Answer from the drawing. Dimensions are ordinates in mm from the lowest x, y and z of the part. A direction names the side the tool comes from. Coordinates: 2 decimals unless noted, no trailing zeros. Order: outer loops, then holes, each group sorted by start corner. A loop starts at its lowest first (then second) coordinate and runs counter-clockwise, first axis right, second up. Notation, with made-up numbers: M 54.5,6.25 L 81.5,6.25 A22 ccw 81.5,37.25 Z; hole C -6.5,13.5 d8. An arc over 180 degrees is marked long. One line per question, with ' | ' between items. Start each with the question number.
1) The mould has two halves that part along X. Classify the marked faces 3, 4, 5 and 6: +X half, -X half, draft (parallel to the pull), parting line (faces both ways), or undercut.
2) Given P1, Ø1.5, axis at y = 1.5, z = 5, coming from the -X side; P2, Ø1.1, axis at y = 1.5, z = 7.5, coming from the +X side (1 decimal); P3, Ø1.5, axis at y = 8, z = 9, coming from the +X side, each flat-ended and moving along its own axis, determine where each tip first touches the part or whether it passes through.
3) Find section D-D, the plane y = 8.5. Write down the section's boundary in (x, z).
4) Find section A-A, the plane x = 5.75. Write down the section's boundary in (y, z) (1 decimal).
5) Consider probe 1 along X at (y, z) = (5, 7); probe 2 along X at (y, z) = (7.5, 8.75) (1 decimal); probe 3 along X at (y, z) = (8.5, 1.25) (1 decimal). Determine where each line is inside the solid, lowest interval first.
6) Find section B-B, the plane y = 5.5. Write down the section's boundary in (x, z).
7) A tool of negligible diameter and unlimited length cuts with its end or side. For the marked faces 1 and 2, from which of +Z, -Z, +X, -X, +Y, -Y can it reach the whole face along a straight path? Write none if from no direction.
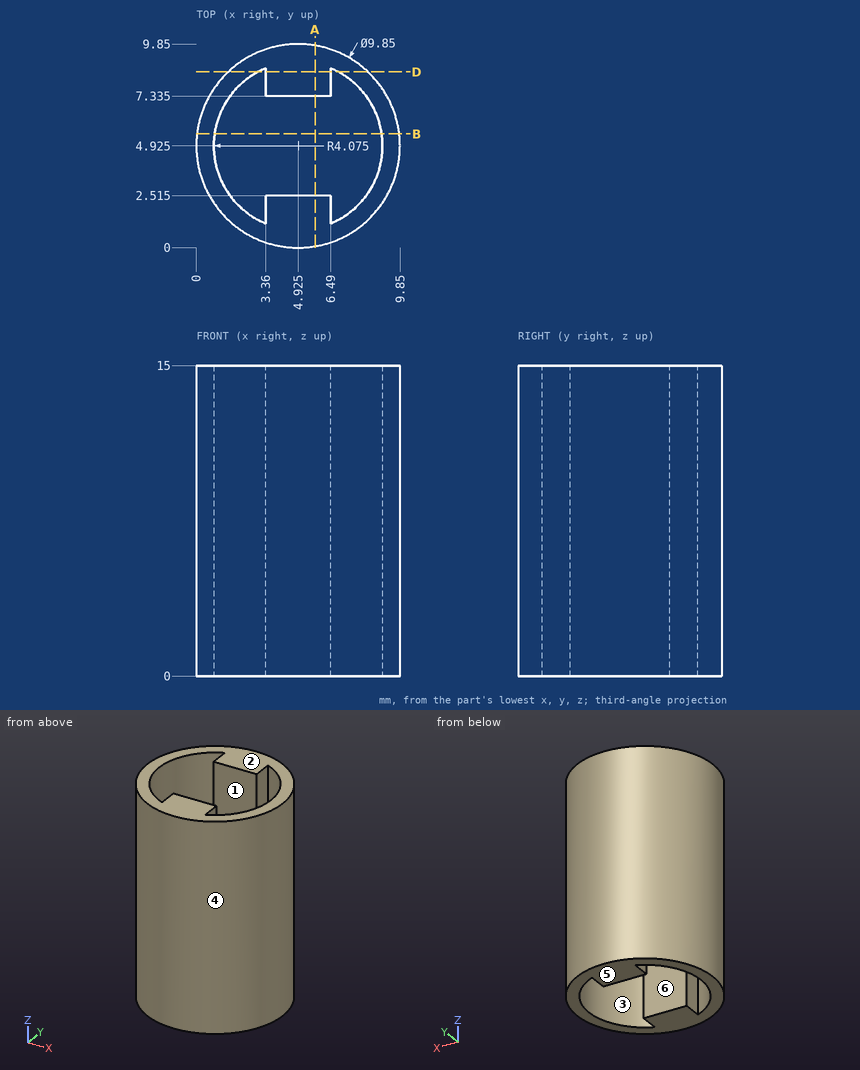
Report:
1) face 3: undercut | face 4: parting line | face 5: draft | face 6: undercut
2) P1: stops at x = 0.79 | P2: stops at x = 8.9 | P3: stops at x = 9.27
3) outline: M 1.54,0 L 2.97,0 L 2.97,15 L 1.54,15 Z; M 3.36,0 L 6.49,0 L 6.49,15 L 3.36,15 Z; M 6.88,0 L 8.31,0 L 8.31,15 L 6.88,15 Z
4) outline: M 0.1,0 L 2.5,0 L 2.5,15 L 0.1,15 Z; M 7.3,0 L 9.8,0 L 9.8,15 L 7.3,15 Z
5) probe 1: x = 0 to 0.85, 9 to 9.85 | probe 2: x = 0.7 to 1.8, 3.4 to 6.5, 8.1 to 9.1 | probe 3: x = 1.5 to 3, 3.4 to 6.5, 6.9 to 8.3
6) outline: M 0.03,0 L 0.89,0 L 0.89,15 L 0.03,15 Z; M 8.96,0 L 9.82,0 L 9.82,15 L 8.96,15 Z
7) face 1: +Z, -Z | face 2: +Z, +X, -X, +Y, -Y
